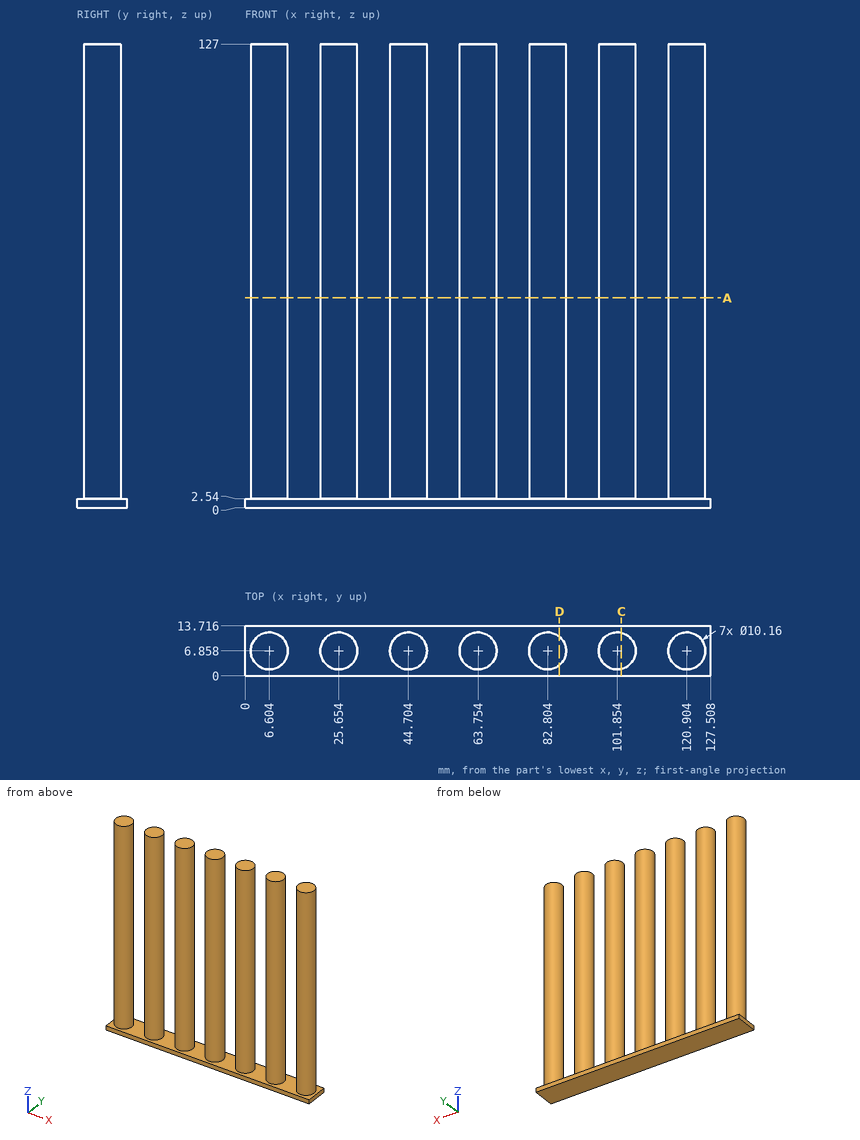
Here's the drawing with two shaded views (mm, measured from the low corner). I have some questions. Coordinates: 2 decimals unless noted, no trailing zeros. Order: outer loops, then holes, each group sorted by start corner. A loop starts at its lowest first (then second) coordinate and runs counter-clockwise, first axis right, second up.
Item 1: If we section it at D-D, the plane x = 86: List the corners of the cut face in (y, z) for me, then the cut area to 3 significant figures.
Response values:
outline: (0, 0) - (13.72, 0) - (13.72, 2.54) - (10.81, 2.54) - (10.81, 127) - (2.91, 127) - (2.91, 2.54) - (0, 2.54) - close
area: 1,020 mm2
Item 2: If we section it at A-A, the plane z = 57.5: List the corners of the cut face in (x, y) for me.
Response values:
outline: circle Ø10.16 at (6.6, 6.86); circle Ø10.16 at (25.65, 6.86); circle Ø10.16 at (44.7, 6.86); circle Ø10.16 at (63.75, 6.86); circle Ø10.16 at (82.8, 6.86); circle Ø10.16 at (101.85, 6.86); circle Ø10.16 at (120.9, 6.86)
Item 3: If we section it at C-C, the plane x = 103: List the corners of the cut face in (y, z) for me, then the cut area to 3 significant figures.
Response values:
outline: (0, 0) - (13.72, 0) - (13.72, 2.54) - (11.81, 2.54) - (11.81, 127) - (1.91, 127) - (1.91, 2.54) - (0, 2.54) - close
area: 1,270 mm2
Item 4: I need wall thicknesses on probe 1 along Z at (x, y) = (14.5, 5.5); probe 2 along Y at (x, z) = (103.5, 17); probe 3 along Y at (x, z) = (45.5, 5). Which ranges of each line are inside material? Lowest first, please.
Response values:
probe 1: z = 0 to 2.54
probe 2: y = 2.05 to 11.66
probe 3: y = 1.84 to 11.88
Item 5: I'm going to push flat-ended pins straight in: pin 1 Ø8 at (x, z) = (50.5, 42) entering from +Y; pin 2 Ø5 at (y, z) = (12, 111.5) entering from -X; pin 3 Ø12 at (x, z) = (44.5, 29) entering from -Y; pin 4 Ø6 at (x, z) = (73, 107.5) entering from +Y. Where does each tip first touch, or does it pass through?
Response values:
pin 1: stops at y = 11.61
pin 2: stops at x = 2.27
pin 3: stops at y = 1.78
pin 4: passes through
